from build123d import *

# Parameters (mm, degrees)
EXTRUDE_1_DEPTH      = 3
SKETCH_28_R          = 12
SKETCH_28_R_2        = 1.5
CUT_EXTRUDE_9_DEPTH  = 4
EXTRUDE_11_DEPTH     = 5
EXTRUDE_14_DEPTH     = 40
CUT_EXTRUDE_12_DEPTH = 4
SKETCH_34_R          = 1.5
CUT_EXTRUDE_13_DEPTH = 4
CHAMFER_1_SIZE       = 2.5
CHAMFER_2_SIZE       = 2.5
CHAMFER_3_SIZE       = 2.5


with BuildPart() as part:
    # 草图1 → 凸台-拉伸1 (new body)
    with BuildSketch(Plane(origin=(0, 0, 0), x_dir=(1, 0, 0), z_dir=(0, 1, 0))):
        with BuildLine():
            Line((-25, 21.381823957), (-25, -28.618176043))
            ThreePointArc((-25, -28.618176043), (0, -38), (25, -28.618176043))
            Line((25, -28.618176043), (25, 21.381823957))
            Line((25, 21.381823957), (-25, 21.381823957))
        make_face()
    extrude(amount=EXTRUDE_1_DEPTH)

    # 草图28 → 切除-拉伸9 (cut)
    with BuildSketch(Plane(origin=(0, 3, 0), x_dir=(1, 0, 0), z_dir=(0, 1, 0))):
        with Locations(Location((0, -3.618176043, 0), (0, 0, 270))):
            Circle(SKETCH_28_R)
        with Locations(Location((-15.5, 11.881823957, 0), (0, 0, 270))):
            Circle(SKETCH_28_R_2)
        with Locations(Location((-15.5, -19.118176043, 0), (0, 0, 270))):
            Circle(SKETCH_28_R_2)
        with Locations(Location((15.5, 11.881823957, 0), (0, 0, 270))):
            Circle(SKETCH_28_R_2)
        with Locations(Location((15.5, -19.118176043, 0), (0, 0, 270))):
            Circle(SKETCH_28_R_2)
    extrude(amount=-CUT_EXTRUDE_9_DEPTH, mode=Mode.SUBTRACT)

    # 草图30 → 凸台-拉伸11 (add)
    with BuildSketch(Plane(origin=(0, 3, 0), x_dir=(1, 0, 0), z_dir=(0, 1, 0))):
        with BuildLine():
            ThreePointArc((-25, -28.618176043), (0, -38), (25, -28.618176043))
            Line((25, -28.618176043), (25, 21.381823957))
            Line((25, 21.381823957), (-25, 21.381823957))
            Line((-25, 21.381823957), (-25, -28.618176043))
        make_face()
        with BuildLine():
            ThreePointArc((23, -27.694764848), (0, -36), (-23, -27.694764848))
            Line((-23, -27.694764848), (-23, 19.381823957))
            Line((-23, 19.381823957), (23, 19.381823957))
            Line((23, 19.381823957), (23, -27.694764848))
        make_face(mode=Mode.SUBTRACT)
    extrude(amount=EXTRUDE_11_DEPTH)

    # 草图32 → 凸台-拉伸14 (add)
    with BuildSketch(Plane.XZ):
        Polygon((-25, -21.381823957), (-25, -9.381823957), (-20, -9.381823957), (-20, -14.381823957), (20, -14.381823957), (20, -10.381823957), (25, -10.381823957), (25, -21.381823957), align=None)
    extrude(amount=EXTRUDE_14_DEPTH)

    # 草图33 → 切除-拉伸12 (cut)
    with BuildSketch(Plane(origin=(0, 0, -21.381823957), x_dir=(-1, 0, 0), z_dir=(0, 0, -1))):
        Polygon((0, -20.330127019), (0, -11.669872981), (-2.5, -11.669872981), (-5, -16), (-2.5, -20.330127019), align=None)
        Polygon((2.5, -11.669872981), (0, -11.669872981), (0, -20.330127019), (2.5, -20.330127019), (5, -16), align=None)
    extrude(amount=-CUT_EXTRUDE_12_DEPTH, mode=Mode.SUBTRACT)

    # 草图34 → 切除-拉伸13 (cut)
    with BuildSketch(Plane(origin=(0, 0, -17.381823957), x_dir=(-1, 0, 0), z_dir=(0, 0, -1))):
        with Locations((0, -16)):
            Circle(SKETCH_34_R)
    extrude(amount=-CUT_EXTRUDE_13_DEPTH, mode=Mode.SUBTRACT)

    # 倒角1
    chamfer_1_edges = [part.edges().sort_by_distance(p)[0] for p in [
        (25, 0, 9.118176043),
    ]]
    chamfer(chamfer_1_edges, length=CHAMFER_1_SIZE)

    # 倒角2
    chamfer_2_edges = [part.edges().sort_by_distance(p)[0] for p in [
        (-25, 0, 9.618176043),
    ]]
    chamfer(chamfer_2_edges, length=CHAMFER_2_SIZE)

    # 倒角3
    chamfer_3_edges = [part.edges().sort_by_distance(p)[0] for p in [
        (0, 0, 38),
    ]]
    chamfer(chamfer_3_edges, length=CHAMFER_3_SIZE)


solid = part.part
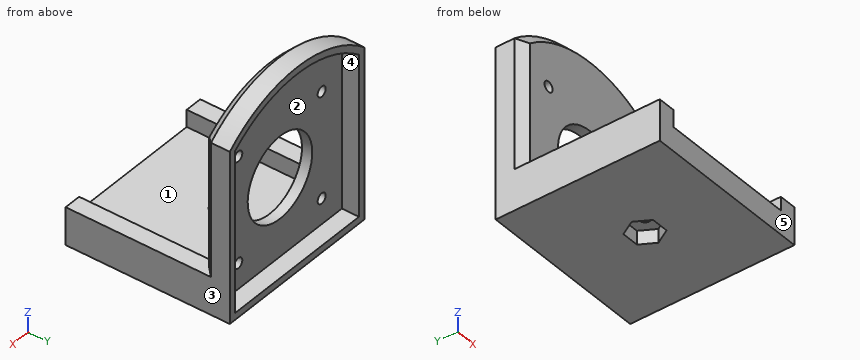
Can you work these out from the model? Positions are in its coordinate system, mm. Face numbers are marked on the shaded views. A direction names the side the tool comes from. Coordinates: 2 decimals unless noted, no trailing zeros. Loops run counter-clockwise (first coordinate to the right, second up) from the corner with the lowest first, then second, coordinate; pieces in that order, holes last. Notation, with made-up numbers: M 60,67 L 85,67 A15 cw 85,72 Z; hole C -26.75,7 d1. An arc over 180 degrees is marked long. Return JSON: item names as keys, results as strings. Group by question number.
Item 1: Imagine slicing it at B-B (z = -3). Please give me the cut outline in (x, y), and give its area (3 significant figures).
Item 2: If I drill on L1, parallel to X at y = 6, z = 27; L2, parallel to X at y = -3, z = -11.5; L3, parallel to Z at x = -15, y = 1, over which ranges is the centre line in solid material (lowest first)? Write a range as from..to.
Item 3: On a 3-axis mill with a long thin cutter (end or side, diameter ignored), from which of +Z, -Z, +X, -X, +Y, -Y can I reach the whole of each face in a straight line? I mean the marked faces 4 and 5. Say none if no direction works.
Item 4: Thinking about a two-plate mould opening in Z: for the marked faces 1, 2 and 3, which applies, released by +Z, released by -Z, zero draft, split by the parting line, or undercut?
Item 5: I'm going to push flat-ended pins straight in: pin 1 Ø5.5 at (x, y) = (-22.5, -29) entering from +Z; pin 2 Ø22.5 at (x, z) = (-1, 1) entering from -Y; pin 3 Ø1.8 at (x, z) = (15.5, 19.12) entering from -Y; pin 4 Ø12 at (x, y) = (6, -16.5) entering from +Z. Where does each tip first touch, or does it pass through?
Item 6: Imagine slicing it at C-C (y = -6.5). Please give me the cut outline in (x, z).
Item 7: Imagine slicing it at D-D (z = 13). Please give me the cut outline in (x, y), and give its area (3 significant figures).
Item 8: Imagine slicing it at A-A (x = 0). Please give me the cut outline in (y, z), and give its area (3 significant figures).
Verdict:
{
 "1": {"outline": "M -25,2.5 L -22.5,0 L -10.01,0 L -10.01,3 L -23,3 L -23,8 L -25,8 Z; M 10.01,0 L 22.5,0 L 25,2.5 L 25,8 L 23,8 L 23,3 L 10.01,3 Z", "area": "104 mm^2"},
 "2": {"L1": "x = -25..-23, 23..25", "L2": "x = -25..-20, 20..25", "L3": "z = -21.38..-13.3, -10.47..17.7, 20.53..33.28"},
 "3": {"face 4": "+Y", "face 5": "+Z, -Z, +X, -X, -Y"},
 "4": {"face 1": "released by +Z", "face 2": "undercut", "face 3": "zero draft"},
 "5": {"pin 1": "stops at z = -9.38", "pin 2": "stops at y = 0", "pin 3": "passes through", "pin 4": "stops at z = -14.38"},
 "6": {"outline": "M -25,-21.38 L 25,-21.38 L 25,-10.38 L 20,-10.38 L 20,-14.38 L -20,-14.38 L -20,-9.38 L -25,-9.38 Z"},
 "7": {"outline": "M -25,2.5 L -22.5,0 L -7.48,0 L -7.48,3 L -23,3 L -23,8 L -25,8 Z; M 7.48,0 L 22.5,0 L 25,2.5 L 25,8 L 23,8 L 23,3 L 7.48,3 Z", "area": "119 mm^2"},
 "8": {"outline": "M -40,-21.38 L -20.33,-21.38 L -20.33,-17.38 L -17.5,-17.38 L -17.5,-14.38 L -40,-14.38 Z; M -14.5,-17.38 L -11.67,-17.38 L -11.67,-21.38 L 8,-21.38 L 8,-19.38 L 3,-19.38 L 3,-8.38 L 0,-8.38 L 0,-14.38 L -14.5,-14.38 Z; M 0,15.62 L 3,15.62 L 3,36 L 8,36 L 8,38 L 2.5,38 L 0,35.5 Z", "area": "359 mm^2"}
}
